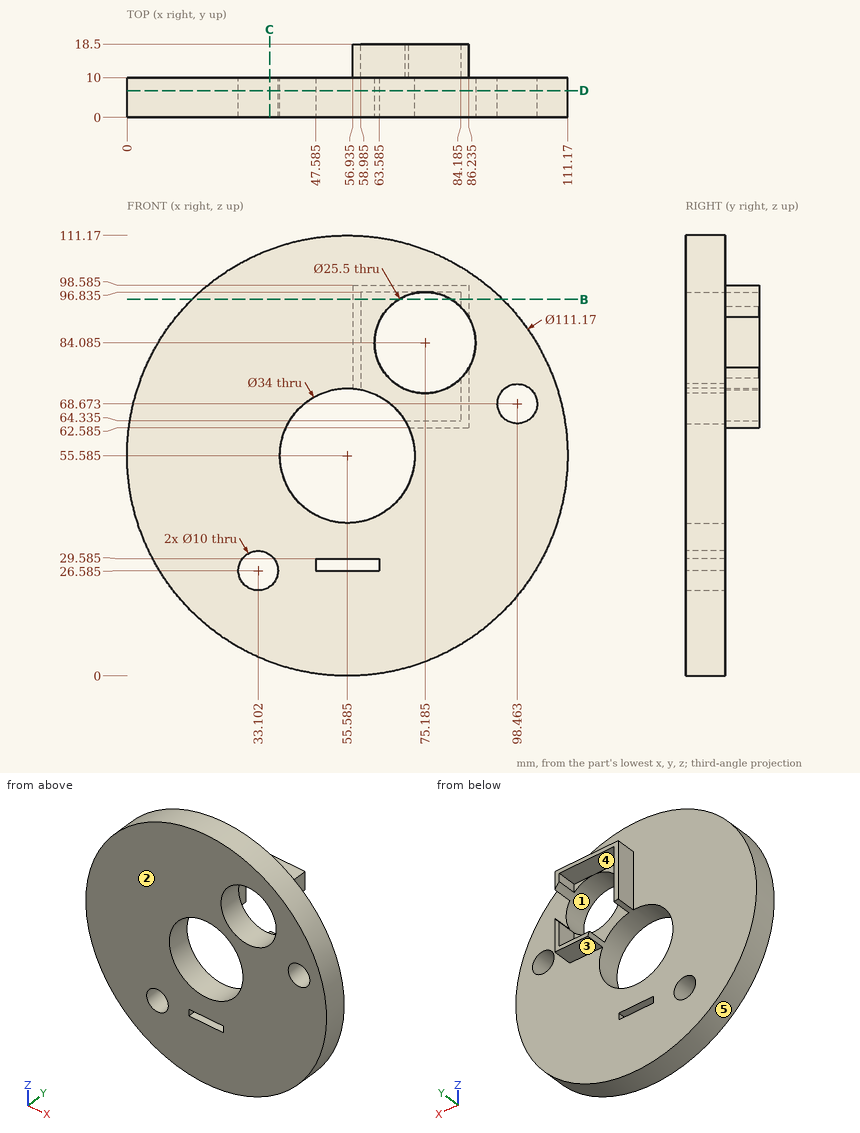
Could you check a few things on this drawing? It's one solid part, dimensions in mm from its lowest x, y, z. A direction names the side the tool comes from. Coordinates: 2 decimals unless noted, no trailing zeros. Order: outer loops, then holes, each group sorted by start corner. A loop starts at its lowest first (then second) coordinate and runs counter-clockwise, first axis right, second up. Notation, with made-up numbers: (40.5, -2.75) -> (65.5, -2.75) arc R20 cw to (65.5, 4.25) -> close; hole circle Ø3 at (-2, 9). An arc over 180 degrees is marked (long way). One line per item, written item: value. Start each with the question number.
1) Imagine slicing it at D-D on y = 6.75. Count the separate pieces of the cut face and the enclosed holes in it, plus the area to 3 significant figures.
2) We'd pull the mould along Z, two halves only. Please class the marked faces 1, 2 and 3: +Z half, -Z half, draft (parallel to the pull), parting line (faces both ways), or undercut.
3) Imagine slicing it at B-B on z = 95. List the corners of the cut face in (x, y) for me (1 decimal).
4) I'm going to push flat-ended pins straight in: pin 1 (7 mm diameter, centred on y = 13, z = 70.5, fed in from +X); pin 2 (7 mm diameter, centred on x = 75, y = 13, fed in from -Z); pin 3 (4 mm diameter, centred on y = 15, z = 95, fed in from +X) (3 decimals). Where does each tip first touch, or does it pass through?
5) If I drill on L1, parallel to Z at x = 58, y = 1.25 (1 decimal); L2, parallel to X at y = 8.75, z = 43.5; L3, parallel to Y at x = 96, z = 29, over which ranges is the centre line in solid material (lowest first)? Write a range as [from, to].
6) Which directions (+Z, -Z, +X, -X, +Y, -Y) give clear straight access to the entire face, cutting with the end or side of a thin tool? Please do the marked faces 4 and 5.
7) Imagine slicing it at C-C on x = 36. List the corners of the cut face in (y, z) for me (1 decimal).
Answer list:
1. separate pieces: 1
1. enclosed holes: 5
1. area: 8,080 mm2
2. face 1: undercut
2. face 2: draft
2. face 3: -Z half
3. outline: (16.4, 0) -> (68.6, 0) -> (68.6, 10) -> (59, 10) -> (59, 18.5) -> (56.9, 18.5) -> (56.9, 10) -> (16.4, 10) -> close; (81.8, 0) -> (94.8, 0) -> (94.8, 10) -> (86.2, 10) -> (86.2, 18.5) -> (84.2, 18.5) -> (84.2, 10) -> (81.8, 10) -> close
4. pin 1: stops at x = 109.6
4. pin 2: stops at z = 2.86
4. pin 3: stops at x = 86.235
5. L1: z = [0.1, 26.6], [29.6, 38.8], [72.4, 111.1]
5. L2: x = [1.33, 43.63], [67.54, 109.84]
5. L3: y = [0, 10]
6. face 4: +Y
6. face 5: +Y, -Y
7. outline: (0, 3.6) -> (10, 3.6) -> (10, 22.5) -> (0, 22.5) -> close; (0, 30.7) -> (10, 30.7) -> (10, 107.6) -> (0, 107.6) -> close
